Source: CAD feature listing. Evaluate the final solid. Frame: model axes, mm. A direction names the side the tool comes from. Round coordinates to 2 decimals unless told otherwise and drop trailing zeros. Write each loop counter-clockwise with the first axis right and the second up, starting at its lowest first coordinate (ties: lowest second). Pieces come first, ordered by that corner, then holes. Notation, with made-up numbers: M 77,-7.75 L 99,-7.75 A14 ccw 99,19.25 Z; hole C -40,22 d2. An arc over 180 degrees is marked long. Use a Markdown table: item, result.
```python
from build123d import *

# Parameters (mm, degrees)
BOSS_EXTRUDE1_DEPTH      = 457.2
BOSS_EXTRUDE1_DEPTH_BACK = 457.2
SKETCH3_W                = 63.5
SKETCH3_H                = 63.5
SKETCH3_W_2              = 50.8
SKETCH3_H_2              = 50.8
SKETCH6_R                = 5.588
CUT_EXTRUDE1_DEPTH       = 463.679319291
SKETCH7_R                = 7.9375
CUT_EXTRUDE2_DEPTH       = 463.679319291


with BuildPart() as part:
    # Sketch3 → Boss-Extrude1 (new, two sides: drawn at the far end of the back side and taken through both)
    with BuildSketch(Plane.XY.offset(-BOSS_EXTRUDE1_DEPTH_BACK)):
        Rectangle(SKETCH3_W, SKETCH3_H)
        Rectangle(SKETCH3_W_2, SKETCH3_H_2, mode=Mode.SUBTRACT)
    extrude(amount=BOSS_EXTRUDE1_DEPTH + BOSS_EXTRUDE1_DEPTH_BACK)

    # Sketch6 → Cut-Extrude1 (cut, through all)
    with BuildSketch(Plane(origin=(0, 31.75, 0), x_dir=(1, 0, 0), z_dir=(0, 1, 0))):
        with Locations(Location((0, 409.575, 0), (0, 0, 270))):
            Circle(SKETCH6_R)
        with Locations(Location((0, -409.575, 0), (0, 0, 270))):
            Circle(SKETCH6_R)
        with Locations(Location((0, -352.425, 0), (0, 0, 270))):
            Circle(SKETCH6_R)
        with Locations(Location((0, 352.425, 0), (0, 0, 270))):
            Circle(SKETCH6_R)
    extrude(amount=-CUT_EXTRUDE1_DEPTH, mode=Mode.SUBTRACT)

    # Sketch7 → Cut-Extrude2 (cut, through all)
    with BuildSketch(Plane(origin=(31.75, 0, 0), x_dir=(0, 0, -1), z_dir=(1, 0, 0))):
        Circle(SKETCH7_R)
    extrude(amount=-CUT_EXTRUDE2_DEPTH, mode=Mode.SUBTRACT)


solid = part.part
```
Q1. Mould query, pull axis Z, two halves, no side actions, for faces 1 (the flat face through (-29, 0, -457.2)), 2 (the cylindrical face through (28.62, -7.75, 1.72)), 3 (the flat face through (0, 25.4, -6)). Classes: +Z half, -Z half, draft (parallel to the pull), parting line (faces both ways), or undercut.
Results are:
| item | result |
|---|---|
| face 1 | -Z half |
| face 2 | undercut |
| face 3 | draft |
Q2. First-contact query: pin 1 Ø18 at (x, z) = (0, -409.575) entering from +Y. Flat tip, straight axial feed; report the tip coordinate or a pass-through.
Results are:
| item | result |
|---|---|
| pin 1 | y = 31.75 |
Q3. Section A-A on z = 0. Return loops of the section in (x, y), plus the area to 3 significant figures.
Results are:
| item | result |
|---|---|
| outline | M -31.75,-31.75 L 31.75,-31.75 L 31.75,-7.94 L 25.4,-7.94 L 25.4,-25.4 L -25.4,-25.4 L -25.4,-7.94 L -31.75,-7.94 Z; M -31.75,7.94 L -25.4,7.94 L -25.4,25.4 L 25.4,25.4 L 25.4,7.94 L 31.75,7.94 L 31.75,31.75 L -31.75,31.75 Z |
| area | 1,250 mm^2 |
Q4. Line query: L1, parallel to Y at x = -23.5, z = 216; L2, parallel to Y at x = 29.25, z = 0. Output: solid intervals per line, ascending.
Results are:
| item | result |
|---|---|
| L1 | -31.75 to -25.4, 25.4 to 31.75 |
| L2 | -31.75 to -7.94, 7.94 to 31.75 |
Q5. Section B-B on y = -17.5. Return loops of the section in (x, z).
Results are:
| item | result |
|---|---|
| outline | M -31.75,-457.2 L -25.4,-457.2 L -25.4,457.2 L -31.75,457.2 Z; M 25.4,-457.2 L 31.75,-457.2 L 31.75,457.2 L 25.4,457.2 Z |
Q6. Reachability of faces 4 (the flat face through (-31.75, 7, -6)), 5 (the flat face through (25.4, 5.3, -6.4)) from +Z, -Z, +X, -X, +Y, -Y: full face, straight path, thin tool, end or side. Return the list, or none.
Results are:
| item | result |
|---|---|
| face 4 | +Z, -Z, -X, +Y, -Y |
| face 5 | +Z, -Z |
